Part model, mm, in its own coordinate system. Give positions to 0.01 mm unless a question says otherwise; leave off trailing zeros. Write each loop counter-clockwise with the first axis right and the second up, starting at its lowest first coordinate (ties: lowest second). Pieces come first, ordered by that corner, then holes. Notation, with made-up numbers: M -35.5,77 L 14.5,77 A16 ccw 14.5,99 Z; hole C 21,52 d9. An arc over 180 degrees is marked long. Use a Markdown table: item, result.
```python
from build123d import *

# Parameters (mm, degrees)
F1_DEPTH = 5
F3_D     = 9
F5_D     = 9


with BuildPart() as f1:
    # F0 (on Front) → F1 (new body)
    with BuildSketch(Plane.XZ):
        Polygon((0, 50), (0, 0), (150, 0), (150, 110), (75, 110), (60, 90), (60, 50), align=None)
    extrude(amount=F1_DEPTH)

    # F3 (through all)
    with Locations(Plane.XZ.offset(5)):
        with Locations((10, 30), (60, 30)):
            Hole(F3_D / 2)

    # F5 (through all)
    with Locations(Plane.XZ.offset(5)):
        with Locations((110, 20), (130, 90)):
            Hole(F5_D / 2)


solid = f1.part
```
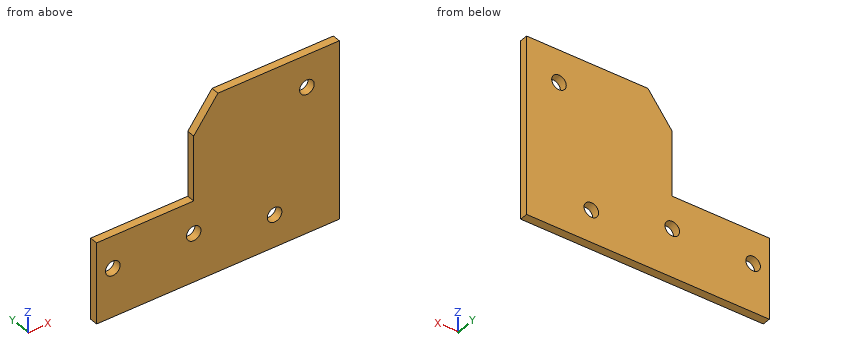
1. Drill centre lines: L1, parallel to Z at x = 110, y = -2.75; L2, parallel to Z at x = 26.5, y = -2.6; L3, parallel to X at y = -4.3, z = 29. Where is each one in solid material? Low to high.
Findings below:
| item | result |
|---|---|
| L1 | 0 to 15.5, 24.5 to 110 |
| L2 | 0 to 50 |
| L3 | 0 to 5.61, 14.39 to 55.61, 64.39 to 150 |
2. Cut at A-A, the plane z = 30. Give the cut face in (x, y).
Findings below:
| item | result |
|---|---|
| outline | M 0,-5 L 5.5,-5 L 5.5,0 L 0,0 Z; M 14.5,-5 L 55.5,-5 L 55.5,0 L 14.5,0 Z; M 64.5,-5 L 150,-5 L 150,0 L 64.5,0 Z |
3. Cut at C-C, the plane y = -1.75. Give the cut face in (x, z).
Findings below:
| item | result |
|---|---|
| outline | M 0,0 L 150,0 L 150,110 L 75,110 L 60,90 L 60,50 L 0,50 Z; hole C 10,30 d9; hole C 60,30 d9; hole C 110,20 d9; hole C 130,90 d9 |
4. Cut at D-D, the plane x = 110. Give the cut face in (y, z).
Findings below:
| item | result |
|---|---|
| outline | M -5,0 L 0,0 L 0,15.5 L -5,15.5 Z; M -5,24.5 L 0,24.5 L 0,110 L -5,110 Z |
5. Cut at B-B, the plane x = 10. Give the cut face in (y, z), then the cut area to 3 significant figures.
Findings below:
| item | result |
|---|---|
| outline | M -5,0 L 0,0 L 0,25.5 L -5,25.5 Z; M -5,34.5 L 0,34.5 L 0,50 L -5,50 Z |
| area | 205 mm2 |
6. Drop flat-ended pins along their axis: P1, Ø1.5, axis at y = -1.5, z = 64.5, coming from the -X side; P2, Ø5.5, axis at x = 130, z = 90, coming from the +Y side; P3, Ø1, axis at x = 67.5, y = -2.5, coming from the +Z side; P4, Ø4, axis at x = 62.5, z = 75.5, coming from the +Y side. Give the stop position or say it passes through.
Findings below:
| item | result |
|---|---|
| P1 | x = 60 |
| P2 | through |
| P3 | z = 100.67 |
| P4 | y = 0 |
